from build123d import *

# Parameters (mm, degrees)
BOSS_EXTRUDE1_DEPTH  = 40
SKETCH2_R            = 11
BOSS_EXTRUDE2_DEPTH  = 2
SKETCH3_R            = 2.5
BOSS_EXTRUDE3_DEPTH  = 22
SKETCH4_R            = 1.5
CUT_EXTRUDE1_DEPTH   = 86.416626016
LPATTERN1_COUNT      = 2
LPATTERN1_PITCH      = 31
LPATTERN1_COUNT_DIR2 = 2
LPATTERN1_PITCH_DIR2 = 31


with BuildPart() as part:
    # Sketch1 → Boss-Extrude1 (new body)
    with BuildSketch(Plane(origin=(0, 0, 0), x_dir=(1, 0, 0), z_dir=(0, 1, 0))):
        Polygon((0, 35), (5, 40), (35, 40), (40, 35), (40, 5), (35, 0), (5, 0), (0, 5), align=None)
    extrude(amount=BOSS_EXTRUDE1_DEPTH)

    # Sketch2 → Boss-Extrude2 (add)
    with BuildSketch(Plane(origin=(0, 40, 0), x_dir=(1, 0, 0), z_dir=(0, 1, 0))):
        with Locations(Location((20, 20, 0), (0, 0, 90))):
            Circle(SKETCH2_R)
    extrude(amount=BOSS_EXTRUDE2_DEPTH)

    # Sketch3 → Boss-Extrude3 (add)
    with BuildSketch(Plane(origin=(0, 42, 0), x_dir=(1, 0, 0), z_dir=(0, 1, 0))):
        with Locations(Location((20, 20, 0), (0, 0, 270))):
            Circle(SKETCH3_R)
    extrude(amount=BOSS_EXTRUDE3_DEPTH)

    # Sketch4 → Cut-Extrude1 (cut, through all)
    with BuildSketch(Plane.XZ):
        with Locations(Location((4.5, -4.5, 0), (0, 0, 270))):
            Circle(SKETCH4_R)
    cut_extrude1 = extrude(amount=-CUT_EXTRUDE1_DEPTH, mode=Mode.SUBTRACT)

    # LPattern1: Cut-Extrude1 2 × 2
    with Locations(*[(i * LPATTERN1_PITCH, 0, -j * LPATTERN1_PITCH_DIR2) for i in range(LPATTERN1_COUNT) for j in range(LPATTERN1_COUNT_DIR2) if (i, j) != (0, 0)]):
        add(cut_extrude1, mode=Mode.SUBTRACT)


solid = part.part
The model under review builds one solid part; all positions refer to its coordinate system, in mm. A direction names the side the tool comes from. Round coordinates to 2 decimals unless told otherwise and drop trailing zeros. Loops run counter-clockwise (first coordinate to the right, second up) from the corner with the lowest first, then second, coordinate; pieces in that order, holes last. Notation, with made-up numbers: (17, 76.25) -> (23, 76.25) arc R31 ccw to (23, 115.25) -> close; hole circle Ø6 at (79.5, 61.25). An arc over 180 degrees is marked (long way). One line per question, with ' | ' between items. Start each with the question number.
Item 1: Machinability: for faces 1 (the face through (40, 20, -20)), 2 (the face through (24.213, 40.986, -30.161)), which of the approach directions +Z, -Z, +X, -X, +Y, -Y give a long, thin tool a straight path to every point of the face, cutting with its end or side? Answer none if there is none.
Item 2: For pin 1 (8 mm diameter, centred on x = 21.5, z = -35, fed in from +Y); pin 2 (11 mm diameter, centred on x = 17, z = -22, fed in from +Y); pin 3 (1.5 mm diameter, centred on y = 30, z = -36, fed in from -X), all flat-tipped, find the tip position at first contact; note any pin that passes through.
Item 3: Add section A-A, the plane y = 23. Write out the cut boundary in (x, z), then the cut area to 3 significant figures.
Item 4: Wall thickness on line 1 along X through (y, z) = (14.5, -4.5); line 2 along X through (y, z) = (30, -35); line 3 along Z through (x, y) = (5.5, 35.5): over which ranges is each line inside the solid? List them lowest first. Write a range as [from, to].
Item 5: Add section B-B, the plane z = -20. Write out the cut boundary in (x, y), then the cut area to 3 significant figures.
Item 6: Add section C-C, the plane x = 20. Write out the cut boundary in (y, z).
Item 7: Draft analysis for pull direction X (two halves, no side actions). For faces 3 (the face through (21.69, 52.85, -21.84)), 4 (the face through (34.17, 19.72, -5.19)), 5 (the face through (20, 20, 0)), state which applies: +X half, -X half, draft (parallel to the pull), parting line (faces both ways), or undercut.
Item 8: Add section D-D, the plane x = 25.5. Write out the cut boundary in (y, z).
Return value:
1) face 1: +Z, -Z, +X, +Y, -Y | face 2: +Y
2) pin 1: stops at y = 40 | pin 2: stops at y = 64 | pin 3: stops at x = 0.25
3) outline: (0, -35) -> (5, -40) -> (35, -40) -> (40, -35) -> (40, -5) -> (35, 0) -> (5, 0) -> (0, -5) -> close; hole circle Ø3 at (4.5, -35.5); hole circle Ø3 at (4.5, -4.5); hole circle Ø3 at (35.5, -35.5); hole circle Ø3 at (35.5, -4.5) | area: 1,520 mm2
4) line 1: x = [0.5, 3], [6, 34], [37, 39.5] | line 2: x = [0, 3.09], [5.91, 34.09], [36.91, 40] | line 3: z = [-40, -36.62], [-34.38, -5.62], [-3.38, 0]
5) outline: (0, 0) -> (40, 0) -> (40, 40) -> (31, 40) -> (31, 42) -> (22.5, 42) -> (22.5, 64) -> (17.5, 64) -> (17.5, 42) -> (9, 42) -> (9, 40) -> (0, 40) -> close | area: 1,750 mm2
6) outline: (0, -40) -> (40, -40) -> (40, -31) -> (42, -31) -> (42, -22.5) -> (64, -22.5) -> (64, -17.5) -> (42, -17.5) -> (42, -9) -> (40, -9) -> (40, 0) -> (0, 0) -> close
7) face 3: parting line | face 4: undercut | face 5: draft
8) outline: (0, -40) -> (40, -40) -> (40, -29.53) -> (42, -29.53) -> (42, -10.47) -> (40, -10.47) -> (40, 0) -> (0, 0) -> close
